Verification items for the finished model (mm, model axes). A direction names the side the tool comes from. Give positions to 0.01 mm unless a question says otherwise; leave off trailing zeros. Loops run counter-clockwise (first coordinate to the right, second up) from the corner with the lowest first, then second, coordinate; pieces in that order, holes last. Notation, with made-up numbers: (44.5, 26) - (50.5, 26) arc R30 cw to (50.5, 52) - close; hole circle Ø5 at (7, 43). An arc over 180 degrees is marked (long way). One line per item, written item: value. Start each with the question number.
1. Sectioned sample at B-B (z = -1). Record the cut outline in (x, y).
2. Scan lines: L1, parallel to Z at x = 8.5, y = 12.5 (3 decimals); L2, parallel to Y at x = 2, z = 0.5; L3, parallel to Y at x = 1.5, z = 2. Record each from-to range of solid material in increasing order. Write a range as [from, to].
3. Mould release check, pull along Y, two halves, no side actions. Record for faces 6 (the flat face through (0, 5, -1)), 7 (the cylindrical face through (4.51, 1.26, 0.17)), 8 (the flat face through (6.826, 20.545, -2.159)): pulls with the +Y half, pulls with the -Y half, needs draft (parallel to the pull), parting line crosses it, or undercut.
4. Sectioned sample at D-D (y = 14). Record the cut outline in (x, z) (3 decimals).
5. Access from +Z, -Z, +X, -X, +Y, -Y to the whole of each face (thin tool, end or side, straight path). Record for faces 1 (the flat face through (4.572, 19, -2)), 2 (the flat face through (5, 11, 0)), 3 (the flat face through (7, 19.001, 0)), 4 (the flat face through (5, 10, -3.175)), 5 (the cylindrical face through (4.51, -2.17, 2.32)).
6. Gauge pin test, flat ends, axial feed: pin 1 (2.5 mm diameter, centred on y = 20.5, z = -1, fed in from -X); pin 2 (1 mm diameter, centred on x = 2, z = -1.5, fed in from +Y); pin 3 (0.6 mm diameter, centred on x = 7, z = 0, fed in from +Y). Record the tip position at first contact, or that the pin passes through.
7. Sectioned sample at C-C (x = 4). Record the cut outline in (y, z) (3 decimals).
from build123d import *

# Parameters (mm, degrees)
SKETCH2_R           = 1.27
BOSS_EXTRUDE1_DEPTH = 9.144
SKETCH3_W           = 4.572
SKETCH3_H           = 3.009435793
CUT_EXTRUDE1_DEPTH  = 25.018241396


with BuildPart() as part:
    # Sketch2 → Boss-Extrude1 (new body)
    with BuildSketch(Plane(origin=(0, 0, 0), x_dir=(0, 0, -1), z_dir=(1, 0, 0))):
        with BuildLine():
            Line((0, 18.415), (0, 3.175))
            ThreePointArc((0, 3.175), (-2.24506403, -2.24506403), (3.175, 0))
            Line((3.175, 0), (3.175, 20.574))
            ThreePointArc((3.175, 20.574), (3.066754835, 20.981875221), (2.770508017, 21.282403148))
            Line((2.770508017, 21.282403148), (1.52985297, 19.787480142))
            Line((1.52985297, 19.787480142), (1.52985297, 19.000960284))
            Line((1.52985297, 19.000960284), (-0.561351088, 19.000960284))
            Line((-0.561351088, 19.000960284), (0, 18.415))
        make_face()
        Circle(SKETCH2_R, mode=Mode.SUBTRACT)
    extrude(amount=BOSS_EXTRUDE1_DEPTH)

    # Sketch3 → Cut-Extrude1 (cut, through all)
    with BuildSketch(Plane(origin=(0, 0, -3.175), x_dir=(-1, 0, 0), z_dir=(0, 0, -1))):
        with Locations((-2.286, 19.777685252)):
            Rectangle(SKETCH3_W, SKETCH3_H)
    extrude(amount=-CUT_EXTRUDE1_DEPTH, mode=Mode.SUBTRACT)


solid = part.part
Results are:
1. outline: (0, -3.01) - (9.14, -3.01) - (9.14, -0.78) - (0, -0.78) - close; (0, 0.78) - (9.14, 0.78) - (9.14, 19) - (4.57, 19) - (4.57, 18.27) - (0, 18.27) - close
2. L1: z = [-3.175, 0]
2. L2: y = [-3.14, -1.17], [1.17, 3.14]
2. L3: y = [-2.47, 2.47]
3. face 6: needs draft
3. face 7: undercut
3. face 8: pulls with the +Y half
4. outline: (0, -3.175) - (9.144, -3.175) - (9.144, 0) - (0, 0) - close
5. face 1: +Z, -Z, -X, +Y
5. face 2: +Z, +X, -X
5. face 3: +Z, +X, -X, +Y
5. face 4: -Z, +X, -X, +Y, -Y
5. face 5: +X, -X
6. pin 1: stops at x = 4.57
6. pin 2: stops at y = 18.27
6. pin 3: stops at y = 19
7. outline: (0, -3.175) - (18.273, -3.175) - (18.273, 0) - (3.175, 0) arc R3.175 ccw (long way) to start; hole circle Ø2.54 at (0, 0)
